Here's how the part is built. I have some questions about the finished solid (model axes, mm). A direction names the side the tool comes from. Round coordinates to 2 decimals unless told otherwise and drop trailing zeros. Write each loop counter-clockwise with the first axis right and the second up, starting at its lowest first coordinate (ties: lowest second). Pieces come first, ordered by that corner, then holes. Notation, with made-up numbers: (89, 78.25) - (138, 78.25) arc R23 cw to (138, 116.25) - close; hole circle Ø5 at (23.25, 64). An arc over 180 degrees is marked (long way). Write item = value, one per line. Start each with the question number.
Item 1: If we section it at C-C (z = 74.75): Please give me the cut outline in (x, y), and give its area (3 significant figures).
Item 2: If I drill on line 1 along Z through (x, y) = (0, 4.5); line 2 along Y through (x, z) = (27, 64.5); line 3 along X through (y, z) = (5.5, -73.5), over which ranges is the centre line in solid material (lowest first)? Write a range as [from, to].
Item 3: If we section it at A-A (y = 28): Please give me the cut outline in (x, z), and give its area (3 significant figures).
Item 4: If we section it at B-B (x = 0): Give the number of separate pieces and of enclosed holes in the cut face, and give its area (3 significant figures).
Item 5: If we section it at D-D (x = 18): Please give me the cut outline in (y, z), and give its area (3 significant figures).
Item 6: Which directions (+Z, -Z, +X, -X, +Y, -Y) give clear straight access to the entire face, cutting with the end or side of a thin tool? Please do faces 4 (the face through (5.6, 28.73, 47.28)), 5 (the face through (-7.14, 28.73, 16.2)), 6 (the face through (-17.827, 15.275, 39.167)), 7 (the face through (-27, 16, 59)), 8 (the face through (-39.477, 28.734, 25.639)).
Item 7: Thinking about a two-plate mould opening in Z: for faces 1 (the face through (-36.199, 32.956, 30.575)), 2 (the face through (1.13, 4.93, 76.52)), 3 (the face through (1, 10, -1)), which applies, pulls with the +Z half, pulls with the -Z half, needs draft (parallel to the pull), parting line crosses it, or undercut?
Item 8: For P1, Ø3.5, axis at x = -64.74, z = 37.37, coming from the +Y side; P2, Ø3, axis at x = -34.5, y = 39.5, coming from the -Z side; P3, Ø2, axis at y = 35, z = 55, coming from the +X side; P4, Ø6, axis at x = 15.5, y = 17.5, coming from the -Z side, each with a flat end and sliding along its axis, tell me the tip position at first contact or that it passes through.
```python
from build123d import *

# Parameters (mm, degrees)
SKETCH1_R                          = 82
BOSS_EXTRUDE5_DEPTH                = 10
TAPPED_HOLE_FOR_M4X0_7_HELICOIL4_D = 4.2
CIRPATTERN5_COUNT                  = 6
BOSS_EXTRUDE7_DEPTH                = 10.7
CUT_EXTRUDE1_DEPTH                 = 137.603415174
BOSS_EXTRUDE8_DEPTH                = 38
BOSS_EXTRUDE9_DEPTH                = 6
CUT_EXTRUDE2_DEPTH                 = 30


with BuildPart() as part:
    # Sketch1 → Boss-Extrude5 (new body)
    with BuildSketch(Plane(origin=(0, 0, 0), x_dir=(1, 0, 0), z_dir=(0, 1, 0))):
        with Locations(Location((0, 0, 0), (0, 0, 270))):
            Circle(SKETCH1_R)
    extrude(amount=BOSS_EXTRUDE5_DEPTH)

    # Tapped Hole for M4x0.7 Helicoil4 (through all)
    with Locations(Plane(origin=(0, 10, 0), x_dir=(1, 0, 0), z_dir=(0, 1, 0))):
        with Locations((0, 74.75)):
            tapped_hole_for_m4x0_7_helicoil4 = Hole(TAPPED_HOLE_FOR_M4X0_7_HELICOIL4_D / 2)

    # CirPattern5: Tapped Hole for M4x0.7 Helicoil4 ×6 about axis
    cirpattern5_axis = Axis((0, 0, 0), (0, 1, 0))
    for i in range(1, CIRPATTERN5_COUNT):
        add(tapped_hole_for_m4x0_7_helicoil4.rotate(cirpattern5_axis, i * 360 / CIRPATTERN5_COUNT), mode=Mode.SUBTRACT)

    # Sketch27 → Boss-Extrude7 (add)
    with BuildSketch(Plane(origin=(0, 10, 0), x_dir=(1, 0, 0), z_dir=(0, 1, 0))):
        Polygon((-44.554655662, -48.436893572), (-27.605576649, -12.205295199), (8.626021723, -29.154374211), (-8.181727906, -65.334302871), align=None)
    extrude(amount=BOSS_EXTRUDE7_DEPTH)

    # Sketch28 → Cut-Extrude1 (cut, through all)
    with BuildSketch(Plane(origin=(18.234649477, 0, 8.471089754), x_dir=(0.4213159772609458, 0, -0.9069139139436854), z_dir=(0.9069139139436853, 0, 0.4213159772609457))):
        Polygon((-62.69968102, 10), (-22.806226852, 20.7), (-62.69968102, 20.7), align=None)
    extrude(amount=-CUT_EXTRUDE1_DEPTH, mode=Mode.SUBTRACT)

    # Sketch14 → Boss-Extrude8 (add)
    with BuildSketch(Plane(origin=(0, 10, 0), x_dir=(1, 0, 0), z_dir=(0, 1, 0))):
        Polygon((-30.130006255, -5.519187558), (-49.089225231, -46.330313685), (-44.554655662, -48.436893572), (-27.605576649, -12.205295199), (8.626021723, -29.154374211), (-8.181727906, -65.334302871), (-3.743529534, -67.396112548), (15.215689442, -26.584986421), align=None)
    extrude(amount=BOSS_EXTRUDE8_DEPTH)

    # Sketch29 → Boss-Extrude9 (add)
    with BuildSketch(Plane(origin=(0, 10, 0), x_dir=(1, 0, 0), z_dir=(0, 1, 0))):
        Polygon((-32.365238615, -57.981021357), (-23.255343874, -62.213114555), (-21.772266919, -59.020681327), (-30.882161661, -54.788588129), align=None)
    extrude(amount=BOSS_EXTRUDE9_DEPTH)

    # Sketch31 → Cut-Extrude2 (cut)
    with BuildSketch(Plane(origin=(-17.964660281, 0, -8.403836988), x_dir=(0.42372697531108894, 0, -0.9057899593138112), z_dir=(0.9057899593138112, 0, 0.42372697531108894))):
        Polygon((-64.82666926, 17.73267596), (-62.752661337, 10), (-62.329980493, 10.1133687), (-62.276430508, 18.416684368), align=None)
    extrude(amount=CUT_EXTRUDE2_DEPTH, mode=Mode.SUBTRACT)


solid = part.part
```
Reply:
q1.outline = (-33.71, 0) - (-2.1, 0) - (-2.1, 10) - (-33.71, 10) - close; (2.1, 0) - (33.71, 0) - (33.71, 10) - (2.1, 10) - close
q1.area = 632 mm2
q2.line_1 = [-82, -76.85], [-72.65, 72.65], [76.85, 82]
q2.line_2 = [0, 10]
q2.line_3 = [-36.36, -1.69], [1.69, 36.36]
q3.outline = (-49.09, 46.33) - (-30.13, 5.52) - (15.22, 26.58) - (-3.74, 67.4) - (-8.18, 65.33) - (8.63, 29.15) - (-27.61, 12.21) - (-44.55, 48.44) - close
q3.area = 650 mm2
q4.separate_pieces = 3
q4.enclosed_holes = 0
q4.area = 2,390 mm2
q5.outline = (0, -80) - (10, -80) - (10, 80) - (0, 80) - close
q5.area = 1,600 mm2
q6.face_4 = +Z, +X, +Y
q6.face_5 = -Z, +X, +Y
q6.face_6 = +Y
q6.face_7 = +Z, -X, +Y
q6.face_8 = -Z, -X, +Y
q7.face_1 = pulls with the +Z half
q7.face_2 = undercut
q7.face_3 = needs draft
q8.P1 = through
q8.P2 = 11.7
q8.P3 = 2.48
q8.P4 = 25.32
